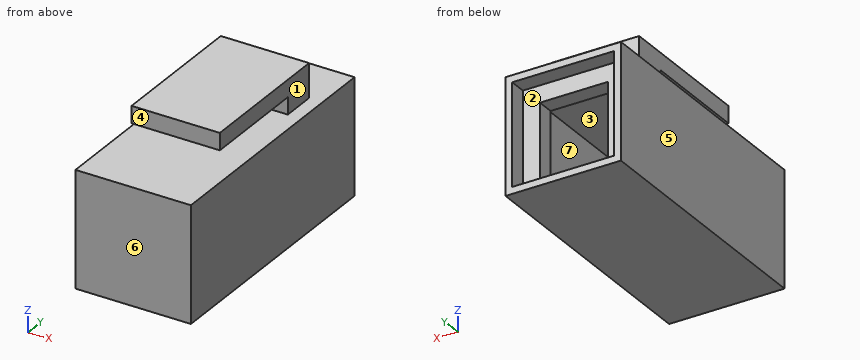
```python
from build123d import *

# Parameters (mm, degrees)
SKETCH1_W           = 34
SKETCH1_H           = 34
SKETCH1_W_2         = 30
SKETCH1_H_2         = 30
BOSS_EXTRUDE1_DEPTH = 75
BOSS_EXTRUDE2_DEPTH = 10
CUT_EXTRUDE1_DEPTH  = 5
SKETCH7_W           = 34
SKETCH7_H           = 34
BOSS_EXTRUDE3_DEPTH = 2
SKETCH8_W           = 26
SKETCH8_H           = 42
BOSS_EXTRUDE4_DEPTH = 10
SKETCH9_W           = 5
SKETCH9_H           = 32.017862038
CUT_EXTRUDE2_DEPTH  = 28


with BuildPart() as part:
    # Sketch1 → Boss-Extrude1 (new body)
    with BuildSketch(Plane(origin=(0, 0, 0), x_dir=(1, 0, 0), z_dir=(0, 1, 0))):
        with Locations((15, -15)):
            Rectangle(SKETCH1_W, SKETCH1_H)
        with Locations((15, -15)):
            Rectangle(SKETCH1_W_2, SKETCH1_H_2, mode=Mode.SUBTRACT)
    extrude(amount=BOSS_EXTRUDE1_DEPTH)

    # Sketch3 → Boss-Extrude2 (add)
    with BuildSketch(Plane(origin=(0, 75, 0), x_dir=(1, 0, 0), z_dir=(0, 1, 0))):
        Polygon((0, 0), (4.981706014, 0), (4.981706014, -25), (24.981706014, -25), (24.981706014, 0), (30, 0), (30, -30), (0, -30), align=None)
    extrude(amount=-BOSS_EXTRUDE2_DEPTH)

    # Sketch4 → Cut-Extrude1 (cut)
    with BuildSketch(Plane(origin=(0, 75, 0), x_dir=(1, 0, 0), z_dir=(0, 1, 0))):
        Polygon((24.981706014, 0), (30.007946467, 0), (30.007946467, -29.950959986), (0, -29.950959986), (0, 0), (4.981706014, 0), (4.981706014, -25), (24.981706014, -25), align=None)
    extrude(amount=-CUT_EXTRUDE1_DEPTH, mode=Mode.SUBTRACT)

    # Sketch7 → Boss-Extrude3 (add)
    with BuildSketch(Plane.XZ):
        with Locations((15, 15)):
            Rectangle(SKETCH7_W, SKETCH7_H)
    extrude(amount=BOSS_EXTRUDE3_DEPTH)

    # Sketch8 → Boss-Extrude4 (add)
    with BuildSketch(Plane.XY.offset(32)):
        with Locations((15, 39)):
            Rectangle(SKETCH8_W, SKETCH8_H)
    extrude(amount=BOSS_EXTRUDE4_DEPTH)

    # Sketch9 → Cut-Extrude2 (cut)
    with BuildSketch(Plane.ZY.offset(-2)):
        with Locations((34.5, 33.991068981)):
            Rectangle(SKETCH9_W, SKETCH9_H)
    extrude(amount=-CUT_EXTRUDE2_DEPTH, mode=Mode.SUBTRACT)


solid = part.part
```
Check sheet for the modelled part. Datum: model origin and axes. Units: mm. Face numbers are marked on the shaded views. A direction names the side the tool comes from. Give positions to 0.01 mm unless a question says otherwise; leave off trailing zeros. Write each loop counter-clockwise with the first axis right and the second up, starting at its lowest first coordinate (ties: lowest second). Pieces come first, ordered by that corner, then holes.
Item 1: Access from +Z, -Z, +X, -X, +Y, -Y to the whole of each face (thin tool, end or side, straight path). Record for the marked faces 1, 2, 3 and 4.
Item 2: Cross-section at C-C (y = 9). Enter the section's corners in (x, z).
Item 3: Cross-section at D-D (z = 26.5). Enter the section's corners in (x, y), and give its area (3 significant figures).
Item 4: Cross-section at A-A (y = 39). Enter the section's corners in (x, z).
Item 5: Draft check along X on the marked faces 5, 6 and 7. Enter one of: released by +X, released by -X, zero draft, split by the parting line, or undercut.
Item 6: Scan lines: L1, parallel to Z at x = 20, y = 46; L2, parallel to X at y = 26, z = 18; L3, parallel to Y at x = 13, z = 28. Record each from-to range of solid material in increasing order.
Item 7: Cross-section at B-B (x = 6). Enter the section's corners in (y, z).
Item 8: Gauge pin test, flat ends, axial feed: pin 1 (4 mm diameter, centred on x = 12.5, z = 19, fed in from +Y); pin 2 (4 mm diameter, centred on x = 12.5, z = 40.5, fed in from -Y); pin 3 (3 mm diameter, centred on x = 3.5, z = 15, fed in from +Y). Record the tip position at first contact, or that the pin passes through.
Report:
1. face 1: +Z, +X, +Y, -Y
1. face 2: +Y
1. face 3: none
1. face 4: +Z, +X, -X, -Y
2. outline: (-2, -2) - (32, -2) - (32, 32) - (-2, 32) - close; hole (0, 0) - (30, 0) - (30, 30) - (0, 30) - close
3. outline: (-2, -2) - (32, -2) - (32, 75) - (30.01, 75) - (30.01, 70) - (0, 70) - (0, 75) - (-2, 75) - close; hole (0, 0) - (30, 0) - (30, 65) - (0, 65) - close
3. area: 518 mm2
4. outline: (-2, -2) - (32, -2) - (32, 32) - (-2, 32) - close; (2, 37) - (28, 37) - (28, 42) - (2, 42) - close; hole (0, 0) - (30, 0) - (30, 30) - (0, 30) - close
5. face 5: released by -X
5. face 6: zero draft
5. face 7: undercut
6. L1: z = -2 to 0, 30 to 32, 37 to 42
6. L2: x = -2 to 0, 30 to 32
6. L3: y = -2 to 0, 65 to 70
7. outline: (-2, -2) - (75, -2) - (75, 0) - (0, 0) - (0, 30) - (65, 30) - (65, 25) - (70, 25) - (70, 29.95) - (75, 29.95) - (75, 32) - (60, 32) - (60, 42) - (18, 42) - (18, 37) - (50, 37) - (50, 32) - (-2, 32) - close
8. pin 1: stops at y = 0
8. pin 2: stops at y = 18
8. pin 3: stops at y = 70
